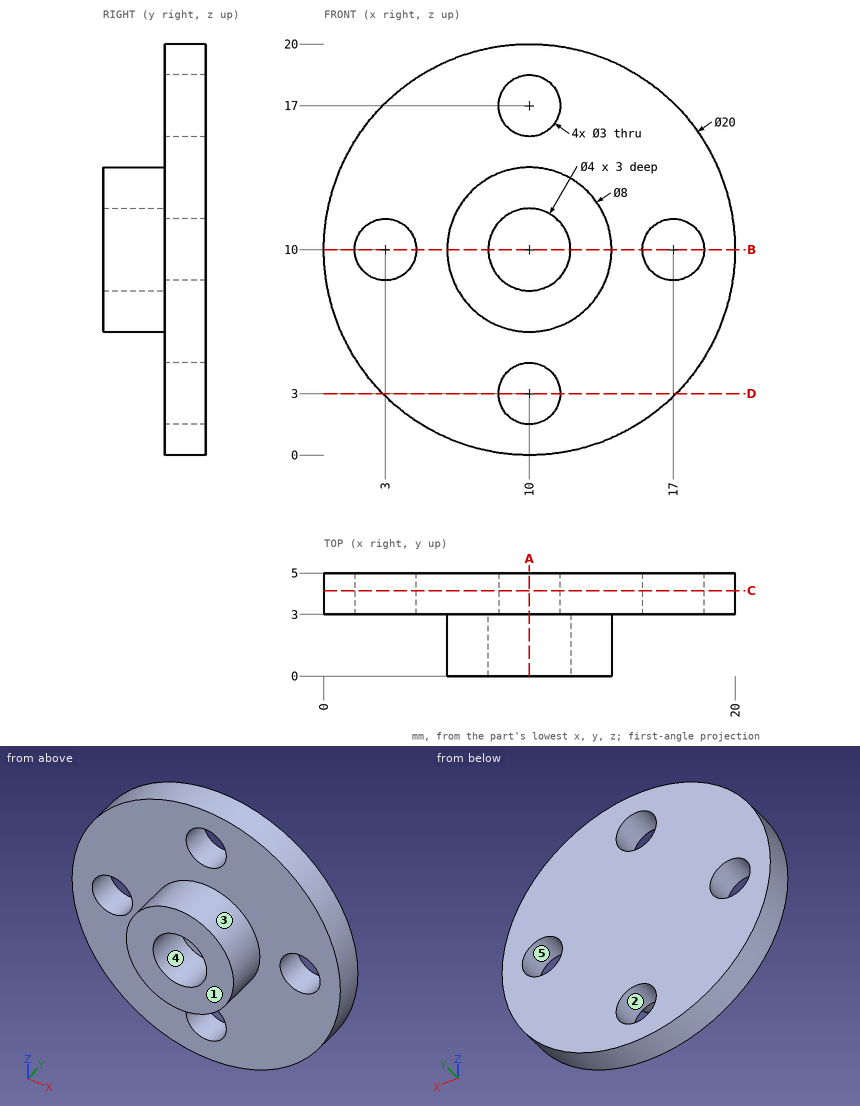
Source: three-view drawing plus pictorial views. Frame: mm from the lowest corner of the part. A direction names the side the tool comes from. Coordinates: 2 decimals unless noted, no trailing zeros. Loops run counter-clockwise (first coordinate to the right, second up) from the corner with the lowest first, then second, coordinate; pieces in that order, holes last. Notation, with made-up numbers: (63.25, -37) -> (104.25, -37) arc R29 cw to (104.25, -11) -> close; hole circle Ø7 at (28.5, 12). An arc over 180 degrees is marked (long way). Answer in a Markdown table with one row per item. Add a question column.
Q1. Section D-D on z = 3. Return the cut outline in (x, y), and give its area (3 significant figures).
Q2. Ray query, line 1 along Z through (x, y) = (10, 3.6); line 2 along Z through (x, y) = (11, 3.25); line 3 along Y through (x, z) = (5.5, 7.75). Return the intervals inside material, ascending.
Q3. Pull-direction query (X, two-part tool) for the marked faces 1, 2 and 3; classes: pulls with the +X half, pulls with the -X half, needs draft (parallel to the pull), parting line crosses it, or undercut.
Q4. Reachability of the marked faces 4 and 5 from +Z, -Z, +X, -X, +Y, -Y: full face, straight path, thin tool, end or side. Return the list, or none.
Q5. Contact query for flat-ended pins moving along their axis: pin 1 Ø2.5 at (x, z) = (10, 3) entering from -Y; pin 2 Ø3 at (x, y) = (13, 0.5) entering from -Z; pin 3 Ø1.5 at (x, y) = (8, 3.5) entering from +Z; pin 4 Ø5 at (x, z) = (10, 17) entering from -Y. Output: stop coordinate, or through.
Q6. Section A-A on x = 10. Return the cut outline in (y, z).
Q7. Section B-B on z = 10. Return the cut outline in (x, y).
Q8. Section C-C on y = 4.15. Return the cut outline in (x, z).
Computed values:
| question | item | result |
|---|---|---|
| 1 | outline | (2.86, 3) -> (8.5, 3) -> (8.5, 5) -> (2.86, 5) -> close; (11.5, 3) -> (17.14, 3) -> (17.14, 5) -> (11.5, 5) -> close |
| 1 | area | 22.6 mm^2 |
| 2 | line 1 | z = 0 to 1.5, 4.5 to 15.5, 18.5 to 20 |
| 2 | line 2 | z = 0.05 to 1.88, 4.12 to 15.88, 18.12 to 19.95 |
| 2 | line 3 | y = 3 to 5 |
| 3 | face 1 | needs draft |
| 3 | face 2 | undercut |
| 3 | face 3 | parting line crosses it |
| 4 | face 4 | -Y |
| 4 | face 5 | +Y, -Y |
| 5 | pin 1 | passes through |
| 5 | pin 2 | stops at z = 6.29 |
| 5 | pin 3 | stops at z = 19.92 |
| 5 | pin 4 | stops at y = 3 |
| 6 | outline | (0, 6) -> (3, 6) -> (3, 4.5) -> (5, 4.5) -> (5, 15.5) -> (3, 15.5) -> (3, 14) -> (0, 14) -> (0, 12) -> (3, 12) -> (3, 8) -> (0, 8) -> close; (3, 0) -> (5, 0) -> (5, 1.5) -> (3, 1.5) -> close; (3, 18.5) -> (5, 18.5) -> (5, 20) -> (3, 20) -> close |
| 7 | outline | (0, 3) -> (1.5, 3) -> (1.5, 5) -> (0, 5) -> close; (4.5, 3) -> (6, 3) -> (6, 0) -> (8, 0) -> (8, 3) -> (12, 3) -> (12, 0) -> (14, 0) -> (14, 3) -> (15.5, 3) -> (15.5, 5) -> (4.5, 5) -> close; (18.5, 3) -> (20, 3) -> (20, 5) -> (18.5, 5) -> close |
| 8 | outline | circle Ø20 at (10, 10); hole circle Ø3 at (3, 10); hole circle Ø3 at (10, 3); hole circle Ø3 at (10, 17); hole circle Ø3 at (17, 10) |
